Autodesk Inventor part; units mm, degrees
ref_plane "YZ Plane" through (0, 0, 0) normal (1, 0, 0) x (0, 1, 0)
ref_plane "XZ Plane" through (0, 0, 0) normal (0, 1, 0) x (-1, 0, 0)
ref_plane "XY Plane" through (0, 0, 0) normal (0, 0, 1) x (1, 0, 0)
sketch "Sketch1" plane through (0, 0, 0) normal (0, 1, 0) x (-1, 0, 0)
  circle A0 centre (0, 0) radius 12.7
  circle A1 centre (0, 0) radius 3.302
  dimension "d0" = 25.4
  dimension "d1" = 6.604
extrude "Extrusion1" add sketch "Sketch1" along normal blind 12.3952
sketch "Sketch2" plane through (0, 12.3952, 0) normal (0, 1, 0) x (1, 0, 0)
  line L0 (0, 0) -> (0, -5.004)
  line L1 (0, -5.004) -> (0, 0)
  line L2 (0, 0) -> (0, 5.004)
  circle A0 centre (0, -5.004) radius 1.0125
  circle A1 centre (0, 5.004) radius 1.0125
  dimension "d4" = 5.004
  dimension "d5" = 5.004
  dimension "d6" = 2.025
  dimension "d7" = 2.025
extrude "Extrusion2" cut sketch "Sketch2" against normal blind 4.445
sketch "Sketch3" plane through (0, 0, 0) normal (0, -1, 0) x (1, 0, 0)
  line L0 (0, 0) -> (0, 5.004)
  line L1 (0, 5.004) -> (0, -5.08)
  circle A0 centre (0, 5.004) radius 1.0125
  line L2 (0, 0) -> (0, -5.004)
  circle A1 centre (0, -5.08) radius 1.0125
  dimension "d10" = 5.004
  dimension "d15" = 2.025
  dimension "d16" = 5.004
  dimension "d17" = 2.025
extrude "Extrusion3" cut sketch "Sketch3" against normal blind 4.445
properties part number "PolarisPost_HeightAdjustment_0p5in_Machined"
For this review, take the finished solid that the model builds, in its own axes (mm). A direction names the side the tool comes from. Give positions to 0.01 mm unless a question says otherwise; leave off trailing zeros. Write each loop counter-clockwise with the first axis right and the second up, starting at its lowest first coordinate (ties: lowest second). Pieces come first, ordered by that corner, then holes. Notation, with made-up numbers: M 68,-26 L 119,-26 A10 cw 119,-9 Z; hole C 43.5,10 d10. An arc over 180 degrees is marked long. Answer as a JSON object with one key per item and string values. Group by question number.
Item 1: Consider section A-A on z = 0. Write out the cut boundary in (x, y), plus the area to 3 significant figures.
Item 2: Tool access review of faces 4 (the flat face through (-3, 12.395, -3)), 5 (the cylindrical face through (-0.132, 2.191, -4.076)), 6 (the flat face through (0, 7.95, 5)): name each direction out of +Z, -Z, +X, -X, +Y, -Y from which nothing blocks a thin tool from reaching the whole face with its end or side.
Item 3: Consider section C-C on y = 6.5. Write out the cut boundary in (x, z), plus the area to 3 significant figures.
Item 4: Consider section D-D on y = 2.75. Write out the cut boundary in (x, z) (1 decimal), plus the area to 3 significant figures.
Item 5: For pin 1 Ø1.2 at (x, z) = (0, 5.004) entering from +Y; pin 2 Ø2 at (x, y) = (6, 9) entering from -Z; pin 3 Ø0.6 at (x, z) = (0, -5) entering from -Y (3 decimals), all flat-tipped, find the tip position at first contact; note any pin that passes through.
Item 6: Consider section B-B on x = 0. Write out the cut boundary in (y, z) (1 decimal), plus the area to 3 significant figures.
Item 7: Draft analysis for pull direction X (two halves, no side actions). For faces 1 (the flat face through (-3, 0, -3)), 2 (the cylindrical face through (2.75, 6.11, 12.4)), 3 (the flat face through (0, 4.445, 5)), state which applies: +X half, -X half, draft (parallel to the pull), parting line (faces both ways), or undercut.
Item 8: For probe 1 along Z at (x, y) = (0, 2.8); probe 2 along Z at (x, y) = (0, 9.95); probe 3 along X at (y, z) = (3.55, -5.08), list the stretches that pass through material, from the lowest coordinate up. Write a range as [from, to].
Check result:
{
 "1": {"outline": "M -12.7,0 L -3.3,0 L -3.3,12.4 L -12.7,12.4 Z; M 3.3,0 L 12.7,0 L 12.7,12.4 L 3.3,12.4 Z", "area": "233 mm^2"},
 "2": {"face 4": "+Z, -Z, +X, -X, +Y", "face 5": "-Y", "face 6": "+Y"},
 "3": {"outline": "C 0,0 d25.4; hole C 0,0 d6.6", "area": "472 mm^2"},
 "4": {"outline": "C 0,0 d25.4; hole C 0,0 d6.6; hole C 0,-5.1 d2; hole C 0,5 d2", "area": "466 mm^2"},
 "5": {"pin 1": "stops at y = 7.95", "pin 2": "stops at z = -11.67", "pin 3": "stops at y = 4.445"},
 "6": {"outline": "M 0,-12.7 L 12.4,-12.7 L 12.4,-6 L 8,-6 L 8,-4 L 12.4,-4 L 12.4,-3.3 L 0,-3.3 L 0,-4.1 L 4.4,-4.1 L 4.4,-6.1 L 0,-6.1 Z; M 0,3.3 L 12.4,3.3 L 12.4,4 L 8,4 L 8,6 L 12.4,6 L 12.4,12.7 L 0,12.7 L 0,6 L 4.4,6 L 4.4,4 L 0,4 Z", "area": "197 mm^2"},
 "7": {"face 1": "draft", "face 2": "parting line", "face 3": "undercut"},
 "8": {"probe 1": "z = [-12.7, -6.09], [-4.07, -3.3], [3.3, 3.99], [6.02, 12.7]", "probe 2": "z = [-12.7, -6.02], [-3.99, -3.3], [3.3, 3.99], [6.02, 12.7]", "probe 3": "x = [-11.64, -1.01], [1.01, 11.64]"}
}
